Can you work these out from the model? Positions are in its coordinate system, mm. A direction names the side the tool comes from. Round coordinates to 2 decimals unless told otherwise and drop trailing zeros. Order: outer loops, then holes, each group sorted by start corner. A loop starts at its lowest first (then second) coordinate and runs counter-clockwise, first axis right, second up.
Autodesk Inventor part; units mm, degrees
ref_plane "YZ Plane" through (0, 0, 0) normal (1, 0, 0) x (0, 1, 0)
ref_plane "XZ Plane" through (0, 0, 0) normal (0, 1, 0) x (-1, 0, 0)
ref_plane "XY Plane" through (0, 0, 0) normal (0, 0, 1) x (1, 0, 0)
sketch "Sketch1" plane through (0, 0, 0) normal (0, 0, 1) x (1, 0, 0)
  line L0 (0, 0) -> (0, 3)
  line L1 (0, 3) -> (25, 3)
  line L2 (25, 3) -> (25, 0)
  line L3 (25, 0) -> (0, 0)
  line L4 (0.5, 3.5) -> (24.5, 3.5)
  line L5 (25, 3) -> (28, 3)
  line L6 (28, 3) -> (28, -17)
  line L7 (28, -17) -> (25, -17)
  line L8 (25, -17) -> (25, 3)
  line L9 (24.5, 3.5) -> (28.5, 3.5)
  line L10 (28.5, 3.5) -> (28.5, -17.5)
  line L11 (28.5, -17.5) -> (24.5, -17.5)
  line L12 (24.5, -17.5) -> (24.5, -0.5)
  line L13 (-3, 3) -> (0, 3)
  line L14 (0, 3) -> (0, -17)
  line L15 (0, -17) -> (-3, -17)
  line L16 (-3, -17) -> (-3, 3)
  line L17 (0.5, 3.5) -> (-3.5, 3.5)
  line L18 (-3.5, 3.5) -> (-3.5, -17.5)
  line L19 (-3.5, -17.5) -> (0.5, -17.5)
  line L20 (24.5, -0.5) -> (0.5, -0.5)
  line L21 (0.5, -17.5) -> (0.5, -0.5)
  line L22 (12.5, 0) -> (12.5, -5.0944) construction
  line L23 (21.5, -3.5) -> (21.5, -20.5)
  line L24 (21.5, -20.5) -> (31.5, -20.5)
  line L25 (31.5, -20.5) -> (31.5, 6.5)
  line L26 (31.5, 6.5) -> (24.5, 6.5)
  line L27 (24.5, 6.5) -> (0.5, 6.5)
  line L28 (0.5, 6.5) -> (-6.5, 6.5)
  line L29 (-6.5, 6.5) -> (-6.5, -20.5)
  line L30 (-6.5, -20.5) -> (3.5, -20.5)
  line L31 (3.5, -20.5) -> (3.5, -3.5)
  line L32 (3.5, -3.5) -> (21.5, -3.5)
  line L33 (21.5, -20.5) -> (3.5, -20.5)
  dimension "d1" = 0.5
  dimension "d3" = 0.5
  dimension "d4" = 0.5
  dimension "d5" = 3
extrude "Extrusion1" add sketch "Sketch1" against normal blind 10 contours L32 L31 L30 L29 L28 L27 L26 L25 L24 L23
extrude "Extrusion2" add sketch "Sketch1" along normal blind 5 contours L14 L15 L16 L13 L0 | L0 L1 L2 L3 | L2 L5 L6 L7 L8 | L4 L9 L10 L11 L12 L20 L21 L19 L18 L17 | L32 L31 L30 L29 L28 L27 L26 L25 L24 L23 | L23 L33 L31 L32
sketch "Sketch2" plane through (3.5, -3.5, -10) normal (0, -1, 0) x (1, 0, 0)
  line L0 (0, 0) -> (-10, 0)
  line L1 (18, 10) -> (18, 0)
  line L2 (0, 0) -> (18, 0) construction
  line L3 (18, 0) -> (18, 10)
  line L4 (18, 10) -> (0, 10) construction
  line L5 (0, 10) -> (0, 0) construction
  point P0 (-3.5, 10)
  point P1 (18, 15)
  point P2 (9, 5)
  dimension "d10" = 5
  dimension "d11" = 9
  dimension "d12" = 10
hole "Hole1" at (12.5, -3.5, -5) direction (0, 1, 0) diameter 5 depth 300 tip angle 118
properties part number "Toper_Carril"
(1) I want a section at B-B, the plane x = 12.5. List the corners of the cut face in (y, z) for me.
(2) I'm going to push flat-ended pins straight in: pin 1 Ø5 at (x, z) = (17, -4) entering from -Y; pin 2 Ø4.5 at (x, z) = (12.5, -5) entering from +Y; pin 3 Ø5 at (x, y) = (17, -12) entering from -Z. Where does each tip first touch, or does it pass through?
(3) I want a section at D-D, the plane z = -4. List the corners of the cut face in (x, y) for me.
(4) I want a section at A-A, the plane z = -0.5. List the corners of the cut face in (x, y) for me, plus the area to 3 significant figures.
(5) On a 3-axis mill with a long thin cutter (end or side, diameter ignored), from which of +Z, -Z, +X, -X, +Y, -Y can I reach the whole of each face in a straight line? I mean faces 4 (the face through (27, -17.5, -5)), 5 (the face through (14.72, -1.98, -6.15)), 6 (the face through (21.5, -12, -5)). Say none if no direction works.
(6) Please list where these lines run through material, in increasing order: probe 1 along X at (y, z) = (-12.75, -8.75); probe 2 along Y at (x, z) = (14.5, -1); probe 3 along X at (y, z) = (5.8, -5).
(7) If we mould it in two halves opening along Y, with no side actions, what happens to faces 1 (the face through (12, -20.5, 1)), 2 (the face through (24.5, -9, -5)), 3 (the face through (14.72, 5.02, -6.15))? For each: pulls with the +Y half, pulls with the -Y half, needs draft (parallel to the pull), parting line crosses it, or undercut.
(8) I want a section at C-C, the plane y = 1.75. List the corners of the cut face in (x, z) for me.
Ans:
1. outline: (-20.5, 0) - (-3.5, 0) - (-3.5, -2.5) - (-0.5, -2.5) - (-0.5, 0) - (3.5, 0) - (3.5, -2.5) - (6.5, -2.5) - (6.5, 5) - (-20.5, 5) - close; (-3.5, -10) - (-0.5, -10) - (-0.5, -7.5) - (-3.5, -7.5) - close; (3.5, -10) - (6.5, -10) - (6.5, -7.5) - (3.5, -7.5) - close
2. pin 1: stops at y = -3.5
2. pin 2: passes through
2. pin 3: stops at z = 0
3. outline: (-6.5, -20.5) - (3.5, -20.5) - (3.5, -3.5) - (10.21, -3.5) - (10.21, -0.5) - (0.5, -0.5) - (0.5, -17.5) - (-3.5, -17.5) - (-3.5, 3.5) - (10.21, 3.5) - (10.21, 6.5) - (-6.5, 6.5) - close; (14.79, -3.5) - (21.5, -3.5) - (21.5, -20.5) - (31.5, -20.5) - (31.5, 6.5) - (14.79, 6.5) - (14.79, 3.5) - (28.5, 3.5) - (28.5, -17.5) - (24.5, -17.5) - (24.5, -0.5) - (14.79, -0.5) - close
4. outline: (-6.5, -20.5) - (3.5, -20.5) - (3.5, -3.5) - (21.5, -3.5) - (21.5, -20.5) - (31.5, -20.5) - (31.5, 6.5) - (-6.5, 6.5) - close; hole (-3.5, -17.5) - (0.5, -17.5) - (0.5, -0.5) - (24.5, -0.5) - (24.5, -17.5) - (28.5, -17.5) - (28.5, 3.5) - (-3.5, 3.5) - close
4. area: 456 mm2
5. face 4: -Z
5. face 5: +Y, -Y
5. face 6: -Z, -Y
6. probe 1: x = -6.5 to -3.5, 0.5 to 3.5, 21.5 to 24.5, 28.5 to 31.5
6. probe 2: y = -3.5 to -0.5, 3.5 to 6.5
6. probe 3: x = -6.5 to 10, 15 to 31.5
7. face 1: pulls with the -Y half
7. face 2: undercut
7. face 3: needs draft
8. outline: (-6.5, -10) - (-3.5, -10) - (-3.5, 0) - (28.5, 0) - (28.5, -10) - (31.5, -10) - (31.5, 5) - (-6.5, 5) - close
